Could you check a few things on this model? Use its own coordinates, in mm. A direction names the side the tool comes from. Give positions to 0.01 mm unless a question says otherwise; leave off trailing zeros. Loops run counter-clockwise (first coordinate to the right, second up) from the corner with the lowest first, then second, coordinate; pieces in that order, holes last. Notation, with made-up numbers: M -19,29 L 9,29 A19 ccw 9,49 Z; hole C -0.75,36.5 d7. An arc over 180 degrees is marked long. Use CSV: the item, a comma, the result in double quotes.
```python
from build123d import *

# Parameters (mm, degrees)
SKETCH_1_R          = 16
SKETCH_1_R_2        = 12.5
EXTRUDE_1_DEPTH     = 4
CHAMFER_1_SIZE      = 0.2
SKETCH_2_R          = 15
SKETCH_2_R_2        = 13.5
CUT_EXTRUDE_1_DEPTH = 0.5
CUT_EXTRUDE_START   = -0.5
SKETCH_3_R          = 15
SKETCH_3_R_2        = 13.5
CUT_EXTRUDE_2_DEPTH = 0.5


with BuildPart() as part:
    # 草图1 → 凸台-拉伸1 (new body)
    with BuildSketch(Plane(origin=(0, 0, 0), x_dir=(1, 0, 0), z_dir=(0, 1, 0))):
        with Locations(Location((0, 0, 0), (0, 0, 270))):
            Circle(SKETCH_1_R)
        with Locations(Location((0, 0, 0), (0, 0, 270))):
            Circle(SKETCH_1_R_2, mode=Mode.SUBTRACT)
    extrude(amount=EXTRUDE_1_DEPTH)

    # 倒角1
    chamfer_1_edges = [part.edges().sort_by_distance(p)[0] for p in [
        (0, 0, -16),
        (0, 4, -16),
        (0, 0, -12.5),
        (0, 4, -12.5),
    ]]
    chamfer(chamfer_1_edges, length=CHAMFER_1_SIZE)

    # 草图2 → 切除-拉伸1 (cut)
    with BuildSketch(Plane(origin=(0, 4, 0), x_dir=(1, 0, 0), z_dir=(0, 1, 0))):
        with Locations(Location((0, 0, 0), (0, 0, 270))):
            Circle(SKETCH_2_R)
        with Locations(Location((0, 0, 0), (0, 0, 270))):
            Circle(SKETCH_2_R_2, mode=Mode.SUBTRACT)
    extrude(amount=-CUT_EXTRUDE_1_DEPTH, mode=Mode.SUBTRACT)

    # 草图3 → 切除-拉伸2 (cut)
    with BuildSketch(Plane.XZ.offset(CUT_EXTRUDE_START)):
        with Locations(Location((0, 0, 0), (0, 0, 90))):
            Circle(SKETCH_3_R)
        with Locations(Location((0, 0, 0), (0, 0, 90))):
            Circle(SKETCH_3_R_2, mode=Mode.SUBTRACT)
    extrude(amount=CUT_EXTRUDE_2_DEPTH, mode=Mode.SUBTRACT)


solid = part.part
```
1. If we mould it in two halves opening along X, with no side actions, what happens to faces 1 (the face through (-5, 0, 12)), 2 (the face through (13.18, 0.25, -2.93)), 3 (the face through (7.85, 3.5, -11.18)), 4 (the face through (-15.62, 1.97, -3.47))? For each: +X half, -X half, draft (parallel to the pull), parting line (faces both ways), or undercut.
Outcome:
face 1,"draft"
face 2,"undercut"
face 3,"undercut"
face 4,"parting line"
2. Which directions (+Z, -Z, +X, -X, +Y, -Y) give clear straight access to the entire face, cutting with the end or side of a thin tool? Please do faces 5 (the face through (-7.85, 0.5, -11.18)), 6 (the face through (-6, 4, 14)), 7 (the face through (0.66, 3.754, -14.985)).
Outcome:
face 5,"-Y"
face 6,"+Z, -Z, +X, -X, +Y"
face 7,"+Y"
3. I'm going to push flat-ended pins straight in: pin 1 Ø2 at (y, z) = (2, -11.5) entering from -X; pin 2 Ø1 at (x, y) = (13, 3) entering from -Z. Where does each tip first touch, or does it pass through?
Outcome:
pin 1,"x = -12.07"
pin 2,"z = -9.99"
4. Please list where these lines run through material, in increasing order: line 1 (X direction, y = 0.2, z = 0); line 2 (X direction, y = 0.3, z = -9.5); line 3 (X direction, y = 2.05, z = 0).
Outcome:
line 1,"-16 to -15, -13.5 to -12.5, 12.5 to 13.5, 15 to 16"
line 2,"-12.87 to -11.61, -9.59 to -8.12, 8.12 to 9.59, 11.61 to 12.87"
line 3,"-16 to -12.5, 12.5 to 16"
5. I want a section at C-C, the plane y = 1.5. List the corners of the cut face in (x, z) for me, then the cut area to 3 significant figures.
Outcome:
outline,"C 0,0 d32; hole C 0,0 d25"
area,"313 mm2"
